```python
from build123d import *

# Parameters (mm, degrees)
MAIN_PLATE_DEPTH                       = 1
HORI_EDGE_DEPTH                        = 117
HORI_EDGE_FILLETS_R                    = 10
M4_CLEARANCE_HOLE1_D                   = 4.5
M4_CLEARANCE_HOLE1_DEPTH               = 178
VERT_EDGE_DEPTH                        = 117
VERT_EDGE_FILLETS_R                    = 10
M4_CLEARANCE_HOLE2_D                   = 4.5
M4_CLEARANCE_HOLE2_DEPTH               = 178
HORI_EDGE_FILLETS_OF_OTHER_HORI_EDGE_R = 10
VERT_EDGE_FILLETS_OF_OTHER_VERT_EDGE_R = 10


# Sheet-metal steps are written as plain solids
with BuildPart() as part:
    # Sketch1 → Main Plate (new body)
    with BuildSketch(Plane.XY):
        Polygon((-86.5, -58.5), (-58.5, -86.5), (58.5, -86.5), (86.5, -58.5), (86.5, 58.5), (58.5, 86.5), (-58.5, 86.5), (-86.5, 58.5), align=None)
    extrude(amount=-MAIN_PLATE_DEPTH)

    # Hori Edge section (across the edge) → Hori Edge (add)
    with BuildSketch(Plane(origin=(-58.5, 88, -1), x_dir=(0, -1, 0), z_dir=(1, 0, 0))):
        with BuildLine():
            Line((-1, 1.5), (-1, 17))
            Line((-1, 17), (0, 17))
            Line((0, 17), (0, 1.5))
            ThreePointArc((0, 1.5), (0.439339828, 0.439339828), (1.5, 0))
            Line((1.5, 0), (1.5, -1))
            ThreePointArc((1.5, -1), (-0.267766953, -0.267766953), (-1, 1.5))
        make_face()
    hori_edge = extrude(amount=HORI_EDGE_DEPTH)

    # Hori Edge Fillets
    hori_edge_fillets_edges = [part.edges().sort_by_distance(p)[0] for p in [
        (-58.5, 88.5, -18),
        (58.5, 88.5, -18),
    ]]
    fillet(hori_edge_fillets_edges, radius=HORI_EDGE_FILLETS_R)

    # M4 Clearance Hole1
    with Locations(Plane(origin=(0, 89, 0), x_dir=(1, 0, 0), z_dir=(0, 1, 0))):
        with Locations((-48.5, 10.042929808), (48.5, 10.042929808)):
            m4_clearance_hole1 = Hole(M4_CLEARANCE_HOLE1_D / 2, depth=M4_CLEARANCE_HOLE1_DEPTH)

    # Vert Edge section (across the edge) → Vert Edge (add)
    with BuildSketch(Plane(origin=(88, 58.5, -1), x_dir=(-1, 0, 0), z_dir=(0, -1, 0))):
        with BuildLine():
            Line((-1, 1.5), (-1, 17))
            Line((-1, 17), (0, 17))
            Line((0, 17), (0, 1.5))
            ThreePointArc((0, 1.5), (0.439339828, 0.439339828), (1.5, 0))
            Line((1.5, 0), (1.5, -1))
            ThreePointArc((1.5, -1), (-0.267766953, -0.267766953), (-1, 1.5))
        make_face()
    vert_edge = extrude(amount=VERT_EDGE_DEPTH)

    # Vert Edge Fillets
    vert_edge_fillets_edges = [part.edges().sort_by_distance(p)[0] for p in [
        (88.5, 58.5, -18),
        (88.5, -58.5, -18),
    ]]
    fillet(vert_edge_fillets_edges, radius=VERT_EDGE_FILLETS_R)

    # M4 Clearance Hole2
    with Locations(Plane(origin=(89, 0, 0), x_dir=(0, 0, -1), z_dir=(1, 0, 0))):
        with Locations((10, 48.5), (10, -48.5)):
            m4_clearance_hole2 = Hole(M4_CLEARANCE_HOLE2_D / 2, depth=M4_CLEARANCE_HOLE2_DEPTH)

    # Other Hori Edge: Hori Edge, M4 Clearance Hole1 across plane
    add(hori_edge.mirror(Plane.ZX))
    add(m4_clearance_hole1.mirror(Plane.ZX), mode=Mode.SUBTRACT)

    # Hori Edge Fillets of Other Hori Edge
    hori_edge_fillets_of_other_hori_edge_edges = [part.edges().sort_by_distance(p)[0] for p in [
        (-58.5, -88.5, -18),
        (58.5, -88.5, -18),
    ]]
    fillet(hori_edge_fillets_of_other_hori_edge_edges, radius=HORI_EDGE_FILLETS_OF_OTHER_HORI_EDGE_R)

    # Other Vert Edge: Vert Edge, M4 Clearance Hole2 across plane
    add(vert_edge.mirror(Plane(origin=(0, 0, 0), x_dir=(0, 0, 1), z_dir=(1, 0, 0))))
    add(m4_clearance_hole2.mirror(Plane(origin=(0, 0, 0), x_dir=(0, 0, 1), z_dir=(1, 0, 0))), mode=Mode.SUBTRACT)

    # Vert Edge Fillets of Other Vert Edge
    vert_edge_fillets_of_other_vert_edge_edges = [part.edges().sort_by_distance(p)[0] for p in [
        (-88.5, 58.5, -18),
        (-88.5, -58.5, -18),
    ]]
    fillet(vert_edge_fillets_of_other_vert_edge_edges, radius=VERT_EDGE_FILLETS_OF_OTHER_VERT_EDGE_R)


solid = part.part
```
Input: part model. Units: mm. Frame: model coordinates. A direction names the side the tool comes from. Coordinates: 2 decimals unless noted, no trailing zeros. Write each loop counter-clockwise with the first axis right and the second up, starting at its lowest first coordinate (ties: lowest second). Pieces come first, ordered by that corner, then holes. Notation, with made-up numbers: (67, 86) - (112, 86) arc R21 ccw to (112, 120) - close; hole circle Ø7 at (-39, 49). An arc over 180 degrees is marked (long way). Put each result on its own line as item: value. Start each with the question number.
1) Reachability of faces 1 (the face through (-1, 1, -1)), 2 (the face through (-1, -88, -10)), 3 (the face through (50.748, -88.493, -10.142)) from +Z, -Z, +X, -X, +Y, -Y: full face, straight path, thin tool, end or side. Return the list, or none.
2) Ray query, L1, parallel to Y at x = -32, z = -11.5; L2, parallel to Y at x = -88.4, z = -10. Return the intervals inside material, ascending.
3) Cut plane A-A (y = -4.5). Return the cut outline in (x, z), plus the area to 3 significant figures.
4) Cut plane D-D (x = 61). Return the cut outline in (y, z), plus the area to 3 significant figures.
5) Contact query for flat-ended pins moving along their axis: pin 1 (3 mm diameter, centred on y = -88.5, z = -5, fed in from -X); pin 2 (3 mm diameter, centred on x = 87, z = -3.5, fed in from +Y); pin 3 (1 mm diameter, centred on x = 51.5, y = 60.5, fed in from -Z); pin 4 (0.8 mm diameter, centred on y = -87.5, z = -2.5, fed in from +X). Output: stop coordinate, or through.
6) Mould query, pull axis Z, two halves, no side actions, for faces 4 (the face through (50.748, 88.493, -10.142)), 5 (the face through (72.3, -72.7, -0.5)), 6 (the face through (88.49, 55.49, -15.15)). Classes: pulls with the +Z half, pulls with the -Z half, needs draft (parallel to the pull), parting line crosses it, or undercut.
7) Cut plane B-B (z = -15.25). Return the cut outline in (x, y).
Resolved:
1. face 1: -Z
1. face 2: -Z, +X, -X
1. face 3: +Y, -Y
2. L1: y = -89 to -88, 88 to 89
2. L2: y = -58.3 to -50.75, -46.25 to 46.25, 50.75 to 58.3
3. outline: (-89, -18) - (-88, -18) - (-88, -2.5) arc R1.5 cw to (-86.5, -1) - (86.5, -1) arc R1.5 cw to (88, -2.5) - (88, -18) - (89, -18) - (89, -2.5) arc R2.5 ccw to (86.5, 0) - (-86.5, 0) arc R2.5 ccw to (-89, -2.5) - close
3. area: 210 mm2
4. outline: (-84, -1) - (84, -1) - (84, 0) - (-84, 0) - close
4. area: 168 mm2
5. pin 1: stops at x = -58.5
5. pin 2: stops at y = 58.5
5. pin 3: stops at z = -1
5. pin 4: passes through
6. face 4: undercut
6. face 5: needs draft
6. face 6: pulls with the -Z half
7. outline: (-89, -55.39) - (-88, -55.39) - (-88, 55.39) - (-89, 55.39) - close; (-55.39, -89) - (55.39, -89) - (55.39, -88) - (-55.39, -88) - close; (-55.39, 88) - (55.39, 88) - (55.39, 89) - (-55.39, 89) - close; (88, -55.39) - (89, -55.39) - (89, 55.39) - (88, 55.39) - close
